Could you check a few things on this model? Use its own coordinates, in mm. A direction names the side the tool comes from. Coordinates: 2 decimals unless noted, no trailing zeros. Order: outer loops, then holes, each group sorted by start corner. A loop starts at its lowest first (then second) coordinate and runs counter-clockwise, first axis right, second up. Notation, with made-up numbers: (-16.5, -22.5) - (28.5, -22.5) arc R26 ccw to (28.5, 3.5) - close; hole circle Ø10 at (51.25, -14.75). An arc over 180 degrees is marked (long way). Answer as a JSON object with one key per item and string values. Group by question number.
(1) Which directions (+Z, -Z, +X, -X, +Y, -Y) give clear straight access to the entire face, cutting with the end or side of a thin tool? Please do faces 4 (the flat face through (-3, -3, 5)), 5 (the cylindrical face through (57.67, -32.3, 18.4)), 6 (the flat face through (27.637, -21.152, 8.028)).
(2) Please list where this line runs through material, in increasing order: probe 1 along X at (y, z) = (-1.5, 1).
(3) Imagine slicing it at B-B, the plane x = 0. Write out the boundary of the cut face in (y, z).
(4) Imagine slicing it at D-D, the plane y = -28.5. Write out the boundary of the cut face in (x, z), and give its area (3 significant figures).
(5) Imagine slicing it at A-A, the plane y = 0. Write out the boundary of the cut face in (x, z), and give its area (3 significant figures).
(6) Will these pins go through, and if not, where does the flat tip stop? P1, Ø2.5, axis at x = 0, y = 2, coming from the +Z side; P2, Ø21.5, axis at x = 14.5, y = -18.5, coming from the +Z side; P3, Ø4.5, axis at x = 60.5, y = -34, coming from the -Z side.
(7) Imagine slicing it at C-C, the plane z = 27.5. Write out the boundary of the cut face in (x, y).
(8) We'd pull the mould along Z, two halves only. Please class faces 1 (the flat face through (32.99, -13.85, 8.03)), 2 (the flat face through (0, 0, 11)), 3 (the flat face through (30, -17, 6)): pulls with the +Z half, pulls with the -Z half, needs draft (parallel to the pull), parting line crosses it, or undercut.
from build123d import *

# Parameters (mm, degrees)
SKETCH1_R                = 3.5
BOSS_EXTRUDE1_DEPTH      = 15
SKETCH2_R                = 4
BOSS_EXTRUDE2_DEPTH      = 5
SKETCH3_R                = 4.5
BOSS_EXTRUDE3_DEPTH      = 5
BOSS_EXTRUDE4_DEPTH      = 4
SKETCH6_R                = 4.5
BOSS_EXTRUDE5_DEPTH      = 1
BOSS_EXTRUDE5_DEPTH_BACK = 5
SKETCH7_R                = 4
BOSS_EXTRUDE6_DEPTH      = 15
SKETCH8_R                = 3.5
BOSS_EXTRUDE7_DEPTH      = 10
FILLET3_R                = 1


with BuildPart() as part:
    # Sketch1 → Boss-Extrude1 (new body)
    with BuildSketch(Plane.XY):
        Circle(SKETCH1_R)
    extrude(amount=-BOSS_EXTRUDE1_DEPTH)

    # Sketch2 → Boss-Extrude2 (add)
    with BuildSketch(Plane.XY):
        Circle(SKETCH2_R)
    extrude(amount=BOSS_EXTRUDE2_DEPTH)

    # Sketch3 → Boss-Extrude3 (add)
    with BuildSketch(Plane.XY.offset(5)):
        Circle(SKETCH3_R)
    extrude(amount=BOSS_EXTRUDE3_DEPTH)

    # Sketch5 → Boss-Extrude4 (add)
    with BuildSketch(Plane.XY.offset(10)):
        with BuildLine():
            Line((0, 0), (-2.25, -3.897114317))
            Line((-2.25, -3.897114317), (58.371778036, -38.897114185))
            ThreePointArc((58.371778036, -38.897114185), (64.518892287, -37.249999982), (62.871778265, -31.102885683))
            Line((62.871778265, -31.102885683), (2.25, 3.897114317))
            Line((2.25, 3.897114317), (0, 0))
        make_face()
    extrude(amount=-BOSS_EXTRUDE4_DEPTH)

    # Sketch6 → Boss-Extrude5 (add, two sides)
    with BuildSketch(Plane.XY.offset(10)) as boss_extrude5_sk:
        Circle(SKETCH6_R)
        with Locations((60.621778036, -34.999999868)):
            Circle(SKETCH6_R)
    extrude(amount=BOSS_EXTRUDE5_DEPTH)
    extrude(boss_extrude5_sk.sketch, amount=-BOSS_EXTRUDE5_DEPTH_BACK)

    # Sketch7 → Boss-Extrude6 (add)
    with BuildSketch(Plane.XY.offset(11)):
        with Locations((60.621778036, -34.999999868)):
            Circle(SKETCH7_R)
    extrude(amount=BOSS_EXTRUDE6_DEPTH)

    # Sketch8 → Boss-Extrude7 (add)
    with BuildSketch(Plane.XY.offset(26)):
        with Locations((60.621778036, -34.999999868)):
            Circle(SKETCH8_R)
    extrude(amount=BOSS_EXTRUDE7_DEPTH)

    # Fillet3
    fillet3_edges = [part.edges().sort_by_distance(p)[0] for p in [
        (-3.5, 0, -15),
        (57.121778036, -34.999999868, 36),
    ]]
    fillet(fillet3_edges, radius=FILLET3_R)


solid = part.part
Result set:
{
 "1": {"face 4": "-Z", "face 5": "+Z", "face 6": "+Z, -Z, -X, -Y"},
 "2": {"probe 1": "x = -3.71 to 3.71"},
 "3": {"outline": "(-5.2, 6) - (-4.5, 6) - (-4.5, 5) - (-4, 5) - (-4, 0) - (-3.5, 0) - (-3.5, -14) arc R1 ccw to (-2.5, -15) - (2.5, -15) arc R1 ccw to (3.5, -14) - (3.5, 0) - (4, 0) - (4, 5) - (4.5, 5) - (4.5, 11) - (-4.5, 11) - (-4.5, 10) - (-5.2, 10) - close"},
 "4": {"outline": "(40.36, 6) - (58.36, 6) - (58.36, 10) - (40.36, 10) - close", "area": "72.0 mm^2"},
 "5": {"outline": "(-4.5, 5) - (-4, 5) - (-4, 0) - (-3.5, 0) - (-3.5, -14) arc R1 ccw to (-2.5, -15) - (2.5, -15) arc R1 ccw to (3.5, -14) - (3.5, 0) - (4, 0) - (4, 5) - (4.5, 5) - (4.5, 6) - (9, 6) - (9, 10) - (4.5, 10) - (4.5, 11) - (-4.5, 11) - close", "area": "217 mm^2"},
 "6": {"P1": "stops at z = 11", "P2": "stops at z = 10", "P3": "stops at z = 5"},
 "7": {"outline": "circle Ø7 at (60.62, -35)"},
 "8": {"face 1": "needs draft", "face 2": "pulls with the +Z half", "face 3": "pulls with the -Z half"}
}
